from build123d import *
from build123d.topology import SkipClean

# Parameters (mm, degrees)
EXTRUDE_START            = 27
SKETCH_2_R               = 12.5
EXTRUDE_1_DEPTH          = 27
EXTRUDE_START_2          = 45
SKETCH_3_R               = 10
EXTRUDE_2_DEPTH          = 45
CUT_EXTRUDE_START        = -8.8
SKETCH_5_OUTSIDE_W       = 83.272
SKETCH_5_OUTSIDE_H       = 83.272
SKETCH_5_OUTSIDE_R       = 11.5
CUT_EXTRUDE_1_DEPTH      = 1.2
CUT_EXTRUDE_START_2      = 7.5
CUT_EXTRUDE_2_DEPTH      = 220.851050141
EXTRUDE_3_REACH          = 293.351
EXTRUDE_START_3          = -64
PATTERN_CIRCULAR_1_COUNT = 6
CHAMFER_1_SIZE           = 2


with BuildPart() as part:
    # 草图1 → 旋转1 (revolve)
    with BuildSketch(Plane.XY):
        with BuildLine():
            Line((0, 0), (0, 10))
            Line((0, 10), (-88.902752641, 10))
            ThreePointArc((-88.902752641, 10), (-94.492922585, 10.633014138), (-99.8, 12.5))
            Line((-99.8, 12.5), (-128.276194705, 12.5))
            ThreePointArc((-128.276194705, 12.5), (-134.192274488, 13.81142246), (-139, 17.5))
            Line((-139, 17.5), (-154, 17.5))
            Line((-154, 17.5), (-154, 0))
            Line((-154, 0), (0, 0))
        make_face()
    revolve(axis=Axis((0, 0, 0), (-1, 0, 0)))

    # 草图2 → 凸台-拉伸1 (add)
    with BuildSketch(Plane.ZY.offset(154).offset(EXTRUDE_START)):
        with Locations(Location((0, 0, 0), (0, 0, 90))):
            Circle(SKETCH_2_R)
    extrude(amount=-EXTRUDE_1_DEPTH)

    # 草图3 → 凸台-拉伸2 (add)
    with BuildSketch(Plane.ZY.offset(181).offset(EXTRUDE_START_2)):
        with Locations(Location((0, 0, 0), (0, 0, 90))):
            Circle(SKETCH_3_R)
    extrude(amount=-EXTRUDE_2_DEPTH)

    # 草图5 outside → 切除-拉伸1 (cut)
    with BuildSketch(Plane.ZY.offset(181).offset(CUT_EXTRUDE_START)):
        Rectangle(SKETCH_5_OUTSIDE_W, SKETCH_5_OUTSIDE_H)
        with Locations(Location((0, 0, 0), (0, 0, 270))):
            Circle(SKETCH_5_OUTSIDE_R, mode=Mode.SUBTRACT)
    extrude(amount=-CUT_EXTRUDE_1_DEPTH, mode=Mode.SUBTRACT)

    # 草图7 → 切除-拉伸2 (cut, through all)
    with BuildSketch(Plane(origin=(0, 0, 0), x_dir=(1, 0, 0), z_dir=(0, 1, 0)).offset(CUT_EXTRUDE_START_2)):
        with BuildLine():
            Line((-226, 3), (-193, 3))
            ThreePointArc((-193, 3), (-190, 0), (-193, -3))
            Line((-193, -3), (-226, -3))
            ThreePointArc((-226, -3), (-229, 0), (-226, 3))
        make_face()
    extrude(amount=CUT_EXTRUDE_2_DEPTH, mode=Mode.SUBTRACT)

    # 草图8 → 凸台-拉伸3 (add, up to next)
    with BuildSketch(Plane(origin=(0, 0, 0), x_dir=(0, 0, -1), z_dir=(1, 0, 0)).offset(EXTRUDE_START_3), mode=Mode.PRIVATE) as extrude_3_sk1:
        with BuildLine():
            Line((12.247448714, 2.5), (9.682458366, 2.5))
            ThreePointArc((9.682458366, 2.5), (10, 0), (9.682458366, -2.5))
            Line((9.682458366, -2.5), (12.247448714, -2.5))
            ThreePointArc((12.247448714, -2.5), (12.5, 0), (12.247448714, 2.5))
        make_face()
    extrude_3_tool1 = extrude(extrude_3_sk1.sketch, amount=-EXTRUDE_3_REACH, mode=Mode.PRIVATE) - part.part
    extrude_3 = extrude_3_tool1.solids().sort_by_distance((-64, 0, -11.154849))[0]
    add(extrude_3)

    # 阵列(圆周)1: 凸台-拉伸3 ×6 about axis
    with SkipClean():  # the faces are left unmerged after this step: merging them gives an invalid solid
        pattern_circular_1_axis = Axis((0, 0, 0), (1, 0, 0))
        for i in range(1, PATTERN_CIRCULAR_1_COUNT):
            add(extrude_3.rotate(pattern_circular_1_axis, i * 360 / PATTERN_CIRCULAR_1_COUNT))

    # 草图9 → 切除-旋转1 (revolve, cut)
    with BuildSketch(Plane(origin=(0, 0, 0), x_dir=(1, 0, 0), z_dir=(0, 1, 0)), mode=Mode.PRIVATE) as cut_revolve_1_sk:
        Polygon((-64, 10), (-64, 12.5), (-66.329579642, 12.5), align=None)
    revolve(cut_revolve_1_sk.sketch.rotate(Axis((0, 0, 0), (1, 0, 0)), 270), axis=Axis((0, 0, 0), (1, 0, 0)), mode=Mode.SUBTRACT)

    # 倒角1
    chamfer_1_edges = [part.edges().sort_by_distance(p)[0] for p in [
        (-226, -10, 0),
        (-181, -12.5, 0),
        (-154, -17.5, 0),
        (0, -10, 0),
    ]]
    chamfer(chamfer_1_edges, length=CHAMFER_1_SIZE)


solid = part.part
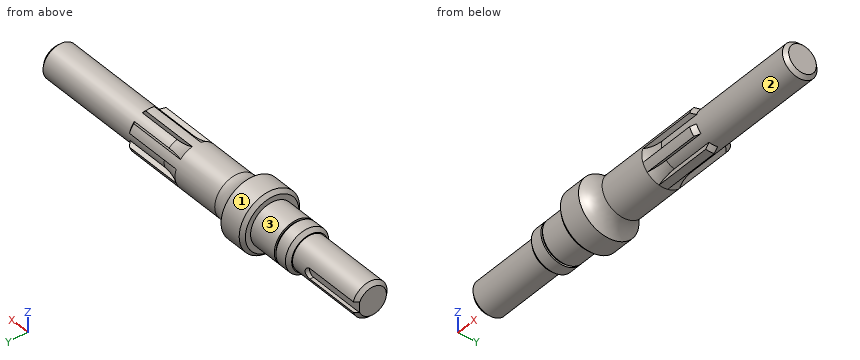
Design review of the part built by this model. Coordinates are the model's own, in mm. Face numbers are marked on the shaded views. A direction names the side the tool comes from. Round coordinates to 2 decimals unless told otherwise and drop trailing zeros. Write each loop counter-clockwise with the first axis right and the second up, starting at its lowest first coordinate (ties: lowest second). Pieces come first, ordered by that corner, then holes.
Item 1: Consider section B-B on x = -147.5. Give the boundary of the cut face in (y, z).
Item 2: For the marked faces 1, 2 and 3, list the 3-axis set-ups (+Z, -Z, +X, -X, +Y, -Y) from which the entire face can be reached by the end or side of a thin tool; tool diameter is ignored.
Item 3: For pin 1 Ø12 at (y, z) = (13.5, -4.5) entering from +X; pin 2 Ø1.6 at (x, y) = (-217, 8.5) entering from -Z; pin 3 Ø8 at (x, y) = (-105, 8.5) entering from +Z; pin 4 Ø5 at (y, z) = (-0.5, -9.5) entering from -X, all flat-tipped, find the tip position at first contact; note any pin that passes through.
Item 4: Wall thickness on L1, parallel to Y at x = -127, z = -0.5; L2, parallel to Y at x = -175.5, z = -5; L3, parallel to X at y = -10, z = 12.5: over which ranges is each line inside the solid? List them lowest first.
Item 5: Consider section A-A on x = -40. Give the boundary of the cut face in (y, z), and give its area (3 significant figures).
Check values:
1. outline: circle Ø35 at (0, 0)
2. face 1: +X, -X
2. face 2: +X
2. face 3: -X
3. pin 1: stops at x = -0.23
3. pin 2: stops at z = -6.38
3. pin 3: stops at z = 11.66
3. pin 4: stops at x = -226
4. L1: y = -12.49 to 12.49
4. L2: y = -11.46 to 11.46
4. L3: x = -153.49 to -137.55
5. outline: circle Ø20 at (0, 0)
5. area: 314 mm2
